Autodesk Inventor part; units mm, degrees
ref_plane "Work Plane2" through (0, 0, 2.5) normal (0, 0, 1) x (1, 0, 0)
ref_plane "Work Plane8" through (0, 0, 0) normal (0.9238795, 0.3826834, 0) x (0, 0, 1)
ref_plane "Work Plane9" through (0, 0, 0) normal (1, 0, 0) x (0, 1, 0)
sketch "Sketch1" plane through (0, 0, 0) normal (0, 0, 1) x (1, 0, 0)
  circle A0 centre (0, 0) radius 10
  dimension "d0" = 20
extrude "Extrusion1" add sketch "Sketch1" along normal blind 5
ref_plane "Work Plane2" through (0, 0, 2.5) normal (0, 0, 1) x (1, 0, 0)
sketch "Sketch2" plane through (0, 0, 0) normal (0, 0, -1) x (-1, 0, 0)
  circle A0 centre (0, 0) radius 10
  circle A1 centre (0, 0) radius 8
  dimension "d3" = 16
surface extrude "Pitch Diameter" sketch "Sketch2" against normal through all shown no curves A1
ref_plane "Work Plane8" through (0, 0, 0) normal (0.9238795, 0.3826834, 0) x (0, 0, 1)
ref_plane "Work Plane9" through (0, 0, 0) normal (1, 0, 0) x (0, 1, 0)
spur gear teeth "Spur Gear" teeth 8 pitch diameter 16 tip diameter 20 root diameter 11 face width 5 start plane through (0, 0, 0) normal (0, 0, -1) x (-1, 0, 0)
sketch "Sketch3" plane through (0, 0, 5) normal (0, 0, 1) x (1, 0, 0)
  circle A0 centre (0, 0) radius 3
  dimension "d49" = 6
extrude "Extrusion2" cut sketch "Sketch3" against normal through all
equation "\"d0\" = da_da"
equation "\"d1\" = da_b"
equation "\"d3\" = da_d"
properties part number "Spur Gear1" material "Steel"
Build history of the part. All positions in model axes, mm. A direction names the side the tool comes from. Round coordinates to 2 decimals unless told otherwise and drop trailing zeros. Write each loop counter-clockwise with the first axis right and the second up, starting at its lowest first coordinate (ties: lowest second). Pieces come first, ordered by that corner, then holes. Notation, with made-up numbers: (-39, 80.25) -> (-26, 80.25) arc R16 ccw to (-26, 104.25) -> close; hole circle Ø7 at (13.5, -30.75). An arc over 180 degrees is marked (long way). Write item = value, one per line.
(1) Band-saw the part on A-A (y = 0). Give the cut face in (x, z).
Answer:
outline = (-10, 0) -> (-3, 0) -> (-3, 5) -> (-10, 5) -> close; (3, 0) -> (10, 0) -> (10, 5) -> (3, 5) -> close
(2) Band-saw the part on D-D (y = 6). Give the cut face in (x, z).
Answer:
outline = (-7.58, 0) -> (-3.65, 0) -> (-3.65, 5) -> (-7.58, 5) -> close; (-1.66, 0) -> (1.66, 0) -> (1.66, 5) -> (-1.66, 5) -> close; (3.65, 0) -> (7.58, 0) -> (7.58, 5) -> (3.65, 5) -> close
(3) Tool access for faces 4 (the face through (-7.614, -1.593, 2.465)), 5 (the face through (-6.511, 4.257, 2.465)), 6 (the face through (4.257, 6.511, 2.465)), 7 (the face through (7.06, 7.08, 2.46)), 8 (the face through (6.511, -4.257, 2.465)): list every direction of +Z, -Z, +X, -X, +Y, -Y with a clear straight run to the whole face (end or side of a thin tool).
Answer:
face_4 = +Z, -Z
face_5 = +Z, -Z, -X
face_6 = +Z, -Z, +Y
face_7 = +Z, -Z, +X, +Y
face_8 = +Z, -Z, +X
(4) Two-plate mould, pull along X, no slides. Class faces 1 (the face through (-7.68, 1.585, 2.465)), 2 (the face through (-2.4, -2.1, 5)), 3 (the face through (10, 0, 2)): pulls with the +X half, pulls with the -X half, needs draft (parallel to the pull), parting line crosses it, or undercut.
Answer:
face_1 = undercut
face_2 = needs draft
face_3 = pulls with the +X half
(5) Flat gauge pins, fed straight in: pin 1 (1.5 mm diameter, centred on y = -1, z = 2.5, fed in from -X); pin 2 (5 mm diameter, centred on x = 0, y = 0, fed in from -Z); pin 3 (1 mm diameter, centred on y = 2.5, z = 1, fed in from +X). Where does each tip first touch, or does it go through?
Answer:
pin_1 = -10
pin_2 = through
pin_3 = 5.34
(6) Probe L1, parallel to Y at x = 0, z = 3.1; L2, parallel to X at y = 6.75, z = 2.6; L3, parallel to Y at x = -7, z = 0.7. List the from-to ranges inside material, lowest first.
Answer:
L1 = -10 to -3, 3 to 10
L2 = -7.38 to -4.58, -1.66 to 1.66, 4.58 to 7.38
L3 = -7.14 to -4.95, -1.65 to 1.65, 4.95 to 7.14
